Input: part model. Units: mm. Frame: model coordinates. A direction names the side the tool comes from. Coordinates: 2 decimals unless noted, no trailing zeros. Write each loop counter-clockwise with the first axis right and the second up, starting at its lowest first coordinate (ties: lowest second). Pieces come first, ordered by that corner, then holes. Notation, with made-up numbers: (3.25, 8.5) - (16.25, 8.5) arc R26 cw to (16.25, 42.5) - close; hole circle Ø3 at (34, 73). An arc over 180 degrees is marked (long way). Use CSV: the item, a comma, the result in double quotes.
```python
from build123d import *

# Parameters (mm, degrees)
EXTRUDE_1_DEPTH     = 12.5
SKETCH_4_W          = 6
SKETCH_4_H          = 43
EXTRUDE_3_DEPTH     = 38
SKETCH_5_W          = 6
SKETCH_5_H          = 13
CUT_EXTRUDE_2_DEPTH = 3
SKETCH_6_W          = 6
SKETCH_6_H          = 43
CUT_EXTRUDE_3_DEPTH = 8
EXTRUDE_5_DEPTH     = 6
FILLET_1_R          = 3
FILLET_2_R          = 3


with BuildPart() as part:
    # 草图1 → 凸台-拉伸1 (new, symmetric)
    with BuildSketch(Plane(origin=(0, 0, 0), x_dir=(1, 0, 0), z_dir=(0, 1, 0))):
        with BuildLine():
            Line((-50, 17.4), (50, 17.4))
            ThreePointArc((50, 17.4), (67.4, 0), (50, -17.4))
            Line((50, -17.4), (-50, -17.4))
            ThreePointArc((-50, -17.4), (-67.4, 0), (-50, 17.4))
        make_face()
        with BuildLine():
            Line((-50, 15.4), (50, 15.4))
            ThreePointArc((50, 15.4), (65.4, 0), (50, -15.4))
            Line((50, -15.4), (-50, -15.4))
            ThreePointArc((-50, -15.4), (-65.4, 0), (-50, 15.4))
        make_face(mode=Mode.SUBTRACT)
    extrude(amount=EXTRUDE_1_DEPTH, both=True)

    # 草图4 → 凸台-拉伸3 (add)
    with BuildSketch(Plane(origin=(0, 12.5, 0), x_dir=(1, 0, 0), z_dir=(0, 1, 0))):
        with Locations((35.717845516, -38.9)):
            Rectangle(SKETCH_4_W, SKETCH_4_H)
    extrude(amount=-EXTRUDE_3_DEPTH)

    # 草图5 → 切除-拉伸2 (cut)
    with BuildSketch(Plane(origin=(0, 0, 17.4), x_dir=(-1, 0, 0), z_dir=(0, 0, -1))):
        with Locations((-35.717845516, -19)):
            Rectangle(SKETCH_5_W, SKETCH_5_H)
    extrude(amount=-CUT_EXTRUDE_2_DEPTH, mode=Mode.SUBTRACT)

    # 草图6 → 切除-拉伸3 (cut)
    with BuildSketch(Plane(origin=(0, 12.5, 0), x_dir=(1, 0, 0), z_dir=(0, 1, 0))):
        with Locations((35.717845516, -38.9)):
            Rectangle(SKETCH_6_W, SKETCH_6_H)
    extrude(amount=-CUT_EXTRUDE_3_DEPTH, mode=Mode.SUBTRACT)

    # 草图8 → 凸台-拉伸5 (add)
    with BuildSketch(Plane.ZY.offset(-32.717845516)):
        Polygon((17.4, 12.5), (17.4, 4.5), (60.4, 4.5), align=None)
    extrude(amount=-EXTRUDE_5_DEPTH)

    # 圆角1
    fillet_1_edges = [part.edges().sort_by_distance(p)[0] for p in [
        (35.717845516, -25.5, 60.4),
        (35.717845516, -25.5, 20.4),
    ]]
    fillet(fillet_1_edges, radius=FILLET_1_R)

    # 圆角2
    fillet_2_edges = [part.edges().sort_by_distance(p)[0] for p in [
        (35.717845516, -12.5, 20.4),
    ]]
    fillet(fillet_2_edges, radius=FILLET_2_R)


solid = part.part
```
(1) Draft query along X for faces 1 (the cylindrical face through (35.76, -24.64, 59.5)), 2 (the flat face through (32.718, -6, 39)), 3 (the flat face through (1, 0, 15.4)). Return one class per face: pulls with the +X half, pulls with the -X half, needs draft (parallel to the pull), parting line crosses it, or undercut.
Check values:
face 1,"needs draft"
face 2,"pulls with the -X half"
face 3,"undercut"
(2) Cut plane B-B on z = 0. Return loops of the section in (x, y), and give its area (3 significant figures).
Check values:
outline,"(-67.4, -12.5) - (-65.4, -12.5) - (-65.4, 12.5) - (-67.4, 12.5) - close; (65.4, -12.5) - (67.4, -12.5) - (67.4, 12.5) - (65.4, 12.5) - close"
area,"100 mm^2"
(3) Cut plane A-A on x = 36.5. Return loops of the section in (y, z).
Check values:
outline,"(-25.5, 23.4) arc R3 ccw to (-22.5, 20.4) - (-15.5, 20.4) arc R3 cw to (-12.5, 17.4) - (-12.5, 15.4) - (12.5, 15.4) - (12.5, 17.4) - (4.5, 60.4) - (-22.5, 60.4) arc R3 ccw to (-25.5, 57.4) - close; (-12.5, -17.4) - (12.5, -17.4) - (12.5, -15.4) - (-12.5, -15.4) - close"
(4) Cut plane D-D on x = -22. Return loops of the section in (y, z).
Check values:
outline,"(-12.5, -17.4) - (12.5, -17.4) - (12.5, -15.4) - (-12.5, -15.4) - close; (-12.5, 15.4) - (12.5, 15.4) - (12.5, 17.4) - (-12.5, 17.4) - close"
(5) Ray query, probe 1 along Z at (x, y) = (23, -6); probe 2 along X at (y, z) = (1.5, 24.5); probe 3 along Z at (x, y) = (-56.5, -1). Return the intervals inside material, ascending. Write a range as from..to.
Check values:
probe 1,"-17.4..-15.4, 15.4..17.4"
probe 2,"32.72..38.72"
probe 3,"-16.14..-13.96, 13.96..16.14"
(6) Cut plane C-C on y = -5. Return loops of the section in (x, z).
Check values:
outline,"(-50, -17.4) - (50, -17.4) arc R17.4 ccw to (50, 17.4) - (38.72, 17.4) - (38.72, 60.4) - (32.72, 60.4) - (32.72, 17.4) - (-50, 17.4) arc R17.4 ccw to start; hole (-50, -15.4) - (50, -15.4) arc R15.4 ccw to (50, 15.4) - (-50, 15.4) arc R15.4 ccw to start"
(7) Reachability of faces 4 (the cylindrical face through (-67.396, 0.175, 0.383)), 5 (the cylindrical face through (65.396, 0.175, -0.339)), 6 (the flat face through (36, -19, 20.4)), 7 (the flat face through (38.718, -6, 39)) from +Z, -Z, +X, -X, +Y, -Y: full face, straight path, thin tool, end or side. Return the list, or none.
Check values:
face 4,"-X, +Y, -Y"
face 5,"+Y, -Y"
face 6,"-Z, +X, -X, -Y"
face 7,"+Z, +X, +Y, -Y"
(8) Pin query (flat end, axial travel): pin 1 Ø2 at (y, z) = (-6.5, 52) entering from -X; pin 2 Ø20 at (x, y) = (-27.5, 0.5) entering from +Z; pin 3 Ø10 at (y, z) = (2.5, -5) entering from -X; pin 4 Ø3 at (x, y) = (35, -20) entering from -Z. Return the tip coordinate at first contact, or that it passes through.
Check values:
pin 1,"x = 32.72"
pin 2,"z = 17.4"
pin 3,"x = -67.4"
pin 4,"z = 20.4"
